Check sheet for the modelled part. Datum: model origin and axes. Units: mm. Give positions to 0.01 mm unless a question says otherwise; leave off trailing zeros. Write each loop counter-clockwise with the first axis right and the second up, starting at its lowest first coordinate (ties: lowest second). Pieces come first, ordered by that corner, then holes. Notation, with made-up numbers: (12, 35) -> (25, 35) arc R29 ccw to (25, 65) -> close; hole circle Ø10 at (-19.5, 88.25). An arc over 180 degrees is marked (long way). Return JSON: item names as keys, results as strings.
from build123d import *

# Parameters (mm, degrees)
F1_DEPTH = 2
F2_R     = 4
F2_W     = 122
F2_H     = 45
F3_DEPTH = 2
F4_R     = 2


with BuildPart() as f1:
    # F0 (on Top) → F1 (new body)
    with BuildSketch(Plane.XY):
        with BuildLine():
            Line((-248, -100), (248, -100))
            ThreePointArc((248, -100), (348, 0), (248, 100))
            Line((248, 100), (-248, 100))
            ThreePointArc((-248, 100), (-348, 0), (-248, -100))
        make_face()
    extrude(amount=F1_DEPTH)

    # F2 (on face) → F3 (cut, through all)
    with BuildSketch(Plane.XY.offset(2)):
        with Locations((318, 0)):
            Circle(F2_R)
        with Locations((-318, 0)):
            Circle(F2_R)
        with Locations((-50, -77.5)):
            Rectangle(F2_W, F2_H)
    extrude(amount=-F3_DEPTH, mode=Mode.SUBTRACT)

    # F4
    f4_edges = [f1.edges().sort_by_distance(p)[0] for p in [
        (11, -55, 1),
        (-111, -55, 1),
    ]]
    fillet(f4_edges, radius=F4_R)


solid = f1.part
(1) Cross-section at A-A on z = 0.5. Enter the section's corners in (x, y).
Reply:
{"outline": "(-248, -100) -> (-111, -100) -> (-111, -57) arc R2 cw to (-109, -55) -> (9, -55) arc R2 cw to (11, -57) -> (11, -100) -> (248, -100) arc R100 ccw to (248, 100) -> (-248, 100) arc R100 ccw to start; hole circle Ø8 at (-318, 0); hole circle Ø8 at (318, 0)"}
(2) Depth check by flat-ended pin: pin 1 Ø1 at (y, z) = (-72.5, 1) entering from +X; pin 2 Ø1 at (y, z) = (64, 1.5) entering from +X. Enter the tip coordinate at first touch or a pass-through.
Reply:
{"pin 1": "x = 317.4", "pin 2": "x = 325.25"}
(3) Cross-section at C-C on y = 76. Enter the section's corners in (x, z), then the cut area to 3 significant figures.
Reply:
{"outline": "(-312.99, 0) -> (312.99, 0) -> (312.99, 2) -> (-312.99, 2) -> close", "area": "1,250 mm^2"}
(4) Cross-section at B-B on x = -20.5. Enter the section's corners in (y, z).
Reply:
{"outline": "(-55, 0) -> (100, 0) -> (100, 2) -> (-55, 2) -> close"}
(5) Thickness scan on L1, parallel to Y at x = -74, z = 0.4; L2, parallel to X at y = -9.5, z = 1.9; L3, parallel to X at y = -18.5, z = 1.1. Record the ranges inside material, lowest first.
Reply:
{"L1": "-55 to 100", "L2": "-347.55 to 347.55", "L3": "-346.27 to 346.27"}
